```python
from build123d import *

# Parameters (mm, degrees)
SKETCH1_W          = 0.25
SKETCH1_H          = 3
SKETCH2_R          = 0.625
CUT_EXTRUDE1_DEPTH = 2


with BuildPart() as part:
    # Sketch1 → Revolve2 (revolve)
    with BuildSketch(Plane(origin=(0, 0, 0), x_dir=(0, 0, -1), z_dir=(1, 0, 0))):
        with Locations((-0.375, 1.5)):
            Rectangle(SKETCH1_W, SKETCH1_H)
        Polygon((0.25, 3), (0, 2.69), (-0.25, 3), (-0.25, 0), (0.25, 0), align=None)
        with Locations((0.375, 1.5)):
            Rectangle(SKETCH1_W, SKETCH1_H)
    revolve(axis=Axis((0, 0, 1.404515092), (0, 0, -1)))

    # Sketch2 → Cut-Extrude1 (cut, through all)
    with BuildSketch(Plane.XY.offset(0.5)):
        Circle(SKETCH2_R)
        with BuildLine():
            ThreePointArc((-2.462019383, 0.434120444), (-2.5, 0), (-2.462019383, -0.434120444))
            ThreePointArc((-2.462019383, -0.434120444), (-2.1724054, -0.636910338), (-1.969615506, -0.347296355))
            ThreePointArc((-1.969615506, -0.347296355), (-2, 0), (-1.969615506, 0.347296355))
            ThreePointArc((-1.969615506, 0.347296355), (-2.1724054, 0.636910338), (-2.462019383, 0.434120444))
        make_face()
        with BuildLine():
            ThreePointArc((-0.684040287, 1.879385242), (-1, 1.732050808), (-1.285575219, 1.532088886))
            ThreePointArc((-1.285575219, 1.532088886), (-1.637783233, 1.562903095), (-1.606969024, 1.915111108))
            ThreePointArc((-1.606969024, 1.915111108), (-1.25, 2.165063509), (-0.855050358, 2.349231552))
            ThreePointArc((-0.855050358, 2.349231552), (-0.534622167, 2.199813433), (-0.684040287, 1.879385242))
        make_face()
        with BuildLine():
            ThreePointArc((1.285575219, 1.532088886), (1, 1.732050808), (0.684040287, 1.879385242))
            ThreePointArc((0.684040287, 1.879385242), (0.534622167, 2.199813433), (0.855050358, 2.349231552))
            ThreePointArc((0.855050358, 2.349231552), (1.25, 2.165063509), (1.606969024, 1.915111108))
            ThreePointArc((1.606969024, 1.915111108), (1.637783233, 1.562903095), (1.285575219, 1.532088886))
        make_face()
        with BuildLine():
            ThreePointArc((1.969615506, -0.347296355), (2, 0), (1.969615506, 0.347296355))
            ThreePointArc((1.969615506, 0.347296355), (2.1724054, 0.636910338), (2.462019383, 0.434120444))
            ThreePointArc((2.462019383, 0.434120444), (2.5, 0), (2.462019383, -0.434120444))
            ThreePointArc((2.462019383, -0.434120444), (2.1724054, -0.636910338), (1.969615506, -0.347296355))
        make_face()
        with BuildLine():
            ThreePointArc((0.684040287, -1.879385242), (1, -1.732050808), (1.285575219, -1.532088886))
            ThreePointArc((1.285575219, -1.532088886), (1.637783233, -1.562903095), (1.606969024, -1.915111108))
            ThreePointArc((1.606969024, -1.915111108), (1.25, -2.165063509), (0.855050358, -2.349231552))
            ThreePointArc((0.855050358, -2.349231552), (0.534622167, -2.199813433), (0.684040287, -1.879385242))
        make_face()
        with BuildLine():
            ThreePointArc((-1.285575219, -1.532088886), (-1, -1.732050808), (-0.684040287, -1.879385242))
            ThreePointArc((-0.684040287, -1.879385242), (-0.534622167, -2.199813433), (-0.855050358, -2.349231552))
            ThreePointArc((-0.855050358, -2.349231552), (-1.25, -2.165063509), (-1.606969024, -1.915111108))
            ThreePointArc((-1.606969024, -1.915111108), (-1.637783233, -1.562903095), (-1.285575219, -1.532088886))
        make_face()
    extrude(amount=-CUT_EXTRUDE1_DEPTH, mode=Mode.SUBTRACT)


solid = part.part
```
Build history of the part. All positions in model axes, mm. A direction names the side the tool comes from. Coordinates: 2 decimals unless noted, no trailing zeros. Order: outer loops, then holes, each group sorted by start corner. A loop starts at its lowest first (then second) coordinate and runs counter-clockwise, first axis right, second up. Notation, with made-up numbers: (-11.5, -30.5) -> (37.5, -30.5) arc R30 cw to (37.5, 4.5) -> close; hole circle Ø4 at (16.25, 1). An arc over 180 degrees is marked (long way). Answer in a Markdown table with one row per item. Add a question column.
Q1. Wall check: line 1 along X through (y, z) = (2.3, -0.15); line 2 along Y through (x, z) = (-1.15, -0.35); line 3 along X through (y, z) = (-1.75, -0.2). Give the ranges that are in metal, low to high. Write a range as [from, to].
Q2. Band-saw the part on A-A, the plane x = 0. List the corners of the cut face in (y, z) (3 decimals), then the cut area to 4 significant figures.
Q3. Drop a flat-ended pin along its axis: pin 1 (1 mm diameter, centred on x = 0, y = 0, fed in from +Z). Give the stop position or say it passes through.
Q4. Band-saw the part on B-B, the plane y = 0. List the corners of the cut face in (x, z) (3 decimals).
Q5. Which spindle directions (+Z, -Z, +X, -X, +Y, -Y) get a long thin tool onto all of the face, cutting with end or side? Do faces 1 (the face through (-1, 0, -0.5)), 2 (the face through (2.5, 0, 0)). Say none if no direction does.
Q6. Band-saw the part on D-D, the plane x = -1.2. Give the number of separate pieces and of enclosed holes in the cut face, then the cut area to 3 significant figures.
Q7. Band-saw the part on C-C, the plane z = -0.1. List the corners of the cut face in (x, y) (3 decimals).
Answers follow:
| question | item | result |
|---|---|---|
| 1 | line 1 | [-1.73, -0.98], [-0.6, 0.6], [0.98, 1.73] |
| 1 | line 2 | [-2.77, -2.22], [-1.64, 1.64], [2.22, 2.77] |
| 1 | line 3 | [-2.36, -1.69], [-0.97, 0.97], [1.69, 2.36] |
| 2 | outline | (-3, -0.5) -> (-0.625, -0.5) -> (-0.625, 0.5) -> (-3, 0.5) -> (-3, 0.25) -> (-2.69, 0) -> (-3, -0.25) -> close; (0.625, -0.5) -> (3, -0.5) -> (3, -0.25) -> (2.69, 0) -> (3, 0.25) -> (3, 0.5) -> (0.625, 0.5) -> close |
| 2 | area | 4.595 mm^2 |
| 3 | pin 1 | through |
| 4 | outline | (-3, -0.5) -> (-2.5, -0.5) -> (-2.5, 0.5) -> (-3, 0.5) -> (-3, 0.25) -> (-2.69, 0) -> (-3, -0.25) -> close; (-2, -0.5) -> (-0.625, -0.5) -> (-0.625, 0.5) -> (-2, 0.5) -> close; (0.625, -0.5) -> (2, -0.5) -> (2, 0.5) -> (0.625, 0.5) -> close; (2.5, -0.5) -> (3, -0.5) -> (3, -0.25) -> (2.69, 0) -> (3, 0.25) -> (3, 0.5) -> (2.5, 0.5) -> close |
| 5 | face 1 | -Z, +X, -X, +Y, -Y |
| 5 | face 2 | +Z, -Z |
| 6 | separate pieces | 3 |
| 6 | enclosed holes | 0 |
| 6 | area | 4.14 mm^2 |
| 7 | outline | circle Ø5.628 at (0, 0); hole (-2.462, -0.434) arc R0.25 ccw to (-1.97, -0.347) arc R2 cw to (-1.97, 0.347) arc R0.25 ccw to (-2.462, 0.434) arc R2.5 ccw to start; hole (-1.607, -1.915) arc R2.5 ccw to (-0.855, -2.349) arc R0.25 ccw to (-0.684, -1.879) arc R2 cw to (-1.286, -1.532) arc R0.25 ccw to start; hole (-1.607, 1.915) arc R0.25 ccw to (-1.286, 1.532) arc R2 cw to (-0.684, 1.879) arc R0.25 ccw to (-0.855, 2.349) arc R2.5 ccw to start; hole circle Ø1.25 at (0, 0); hole (0.684, -1.879) arc R0.25 ccw to (0.855, -2.349) arc R2.5 ccw to (1.607, -1.915) arc R0.25 ccw to (1.286, -1.532) arc R2 cw to start; hole (0.684, 1.879) arc R2 cw to (1.286, 1.532) arc R0.25 ccw to (1.607, 1.915) arc R2.5 ccw to (0.855, 2.349) arc R0.25 ccw to start; hole (1.97, -0.347) arc R0.25 ccw to (2.462, -0.434) arc R2.5 ccw to (2.462, 0.434) arc R0.25 ccw to (1.97, 0.347) arc R2 cw to start |
